Here's how the part is built. I have some questions about the finished solid (model axes, mm). Face numbers are marked on the shaded views. A direction names the side the tool comes from. Coordinates: 2 decimals unless noted, no trailing zeros. Loops run counter-clockwise (first coordinate to the right, second up) from the corner with the lowest first, then second, coordinate; pieces in that order, holes last. Notation, with made-up numbers: (88.5, 23.5) -> (94.5, 23.5) arc R14 cw to (94.5, 41.5) -> close; hole circle Ø7 at (-28, 12.5). An arc over 180 degrees is marked (long way). Answer as a JSON object with one key per item and string values. Group by question number.
Q1. I want a section at A-A on y = -8. Write out the boundary of the cut face in (x, z), then the cut area to 3 significant figures.
Q2. I'm going to push flat-ended pins straight in: pin 1 (1.2 mm diameter, centred on y = 3.5, z = 3, fed in from -X); pin 2 (0.8 mm diameter, centred on x = 5.5, z = 2.5, fed in from +Y); pin 3 (1.2 mm diameter, centred on y = -6.5, z = 3.5, fed in from +X). Where does each tip first touch, or does it pass through?
Q3. I need wall thicknesses on line 1 (X direction, y = -12, z = 2.05); line 2 (X direction, y = -19.45, z = 2.5); line 3 (Y direction, x = 5, z = 3.65). Which ranges of each line are inside material? Lowest first, please.
Q4. On a 3-axis mill with a long thin cutter (end or side, diameter ignored), from which of +Z, -Z, +X, -X, +Y, -Y can I reach the whole of each face in a straight line? I mean the marked faces 4, 5 and 6. Say none if no direction works.
Q5. Thinking about a two-plate mould opening in X: for the marked faces 1, 2 and 3, which applies, released by +X, released by -X, zero draft, split by the parting line, or undercut?
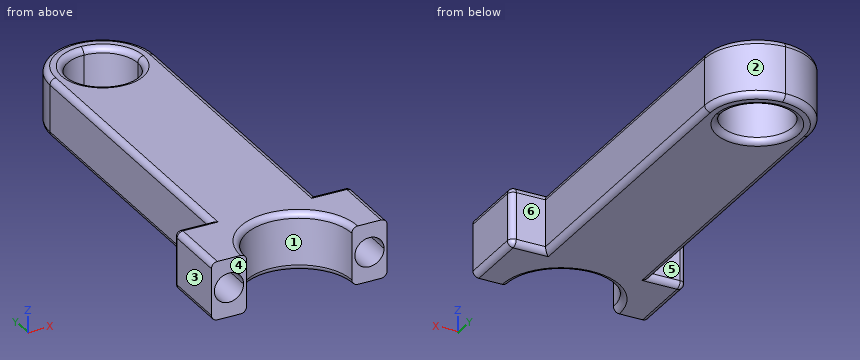
```python
from build123d import *

# Parameters (mm, degrees)
F1_DEPTH = 5
F2_R     = 4.49999
F3_R     = 0.5
F5_DEPTH = 5


# Not quite as in the source:
# - a fillet or chamfer is up to 0.001 mm smaller than in the source, because OpenCascade refuses the exact size
# - a feature names something its author has since deleted; it is built from what else it names


with BuildPart() as f1:
    # F0 (on Top) → F1 (new body)
    with BuildSketch(Plane.XY):
        with BuildLine():
            Line((4.5, -14.8228148893), (-4.5, -14.8228148893))
            Line((-4.5, -14.8228148893), (-7.5, -14.8228148893))
            Line((-7.5, -14.8228148893), (-7.5, -20.8228148893))
            Line((-7.5, -20.8228148893), (-4.5, -20.8228148893))
            ThreePointArc((-4.5, -20.8228148893), (0, -16.3228148893), (4.5, -20.8228148893))
            Line((4.5, -20.8228148893), (7.5, -20.8228148893))
            Line((7.5, -20.8228148893), (7.5, -14.8228148893))
            Line((7.5, -14.8228148893), (4.5, -14.8228148893))
        make_face()
        Polygon((0, 15.1771851107), (-4.5, 15.1771851107), (-4.5, -14.8228148893), (4.5, -14.8228148893), (4.5, 15.1771851107), align=None)
        with BuildLine():
            ThreePointArc((3, 10.6771851107), (-2.1213203436, 8.5558647672), (0, 13.6771851107))
            ThreePointArc((0, 13.6771851107), (2.1213203436, 12.7985054543), (3, 10.6771851107))
        make_face(mode=Mode.SUBTRACT)
    extrude(amount=F1_DEPTH)

    # F2 (radius 4.5 in the source; OpenCascade refuses exactly that, so slightly less here)
    f2_edges = [f1.edges().sort_by_distance(p)[0] for p in [
        (4.5, 15.177185, 2.5),
        (-4.5, 15.177185, 2.5),
    ]]
    fillet(f2_edges, radius=F2_R)

    # F3
    f3_edges = [f1.edges().sort_by_distance(p)[0] for p in [
        (-4.5, -2.07281, 5),
        (-4.5, -2.07281, 0),
        (-6, -14.822815, 5),
        (-6, -14.822815, 0),
        (-7.5, -14.822815, 2.5),
        (7.5, -14.822815, 2.5),
        (6, -14.822815, 0),
        (6, -14.822815, 5),
        (-7.5, -17.822815, 0),
        (-7.5, -17.822815, 5),
        (7.5, -17.822815, 5),
        (7.5, -17.822815, 0),
        (-3, 10.677185, 5),
        (-3, 10.677185, 0),
        (0, -16.322815, 5),
        (0, -16.322815, 0),
        (4.5, -2.07281, 0),
        (4.5, -2.07281, 5),
        (3.181983, 13.859169, 0),
        (0, 15.177185, 0),
        (-3.181983, 13.859169, 0),
        (3.181983, 13.859169, 5),
        (0, 15.177185, 5),
        (-3.181983, 13.859169, 5),
    ]]
    fillet(f3_edges, radius=F3_R)

    # F4 (on face) → F5 (cut)
    with BuildSketch(Plane.XZ.offset(20.8228148893)):
        with BuildLine():
            ThreePointArc((7.25, 2.5), (6.8838834765, 3.3838834765), (6, 3.75))
            Line((6, 3.75), (6, 2.5))
            Line((6, 2.5), (4.75, 2.5))
            ThreePointArc((4.75, 2.5), (6, 1.25), (7.25, 2.5))
        make_face()
        with BuildLine():
            Line((6, 2.5), (6, 3.75))
            ThreePointArc((6, 3.75), (5.1161165235, 3.3838834765), (4.75, 2.5))
            Line((4.75, 2.5), (6, 2.5))
        make_face()
        with BuildLine():
            Line((-6, 2.5), (-6, 3.75))
            ThreePointArc((-6, 3.75), (-6.8838834765, 1.6161165235), (-4.75, 2.5))
            Line((-4.75, 2.5), (-6, 2.5))
        make_face()
        with BuildLine():
            ThreePointArc((-4.75, 2.5), (-5.1161165235, 3.3838834765), (-6, 3.75))
            Line((-6, 3.75), (-6, 2.5))
            Line((-6, 2.5), (-4.75, 2.5))
        make_face()
    extrude(amount=-F5_DEPTH, mode=Mode.SUBTRACT)


solid = f1.part
```
Result set:
{
 "1": {"outline": "(-4.5, 0.5) arc R0.5 ccw to (-4, 0) -> (4, 0) arc R0.5 ccw to (4.5, 0.5) -> (4.5, 4.5) arc R0.5 ccw to (4, 5) -> (-4, 5) arc R0.5 ccw to (-4.5, 4.5) -> close", "area": "44.8 mm²"},
 "2": {"pin 1": "stops at x = -4.5", "pin 2": "stops at y = -14.82", "pin 3": "stops at x = 4.5"},
 "3": {"line 1": "x = -4.5 to 4.5", "line 2": "x = -7.5 to -7.25, -4.75 to -4.29, 4.29 to 4.75, 7.25 to 7.5", "line 3": "y = -20.82 to -14.82"},
 "4": {"face 4": "+Z, -Z, +X, -X, -Y", "face 5": "+Z, -Z, -X, +Y", "face 6": "+Z, -Z, +X, +Y"},
 "5": {"face 1": "undercut", "face 2": "released by +X", "face 3": "released by -X"}
}
